from build123d import *

# Parameters (mm, degrees)
F1_DEPTH    = 15
F3_DEPTH    = 65
F4_T1_DEPTH = 15
F4_T3_DEPTH = 80
F4_T8_DEPTH = 80


# Not quite as in the source:
# - a fillet or chamfer that OpenCascade refuses, or shapes differently, is made with other operations: its cross-section is extruded or revolved along the edge and cut away or added
# - a feature names something its author has since deleted; it is built from what else it names


with BuildPart() as f1:
    # F0 (on Top) → F1 (new body)
    with BuildSketch(Plane.XY):
        Polygon((0, 88), (0, 0), (18, 0), (18, 5), (14, 5), (14, 4), (4, 4), (4, 84), (14, 84), (17, 81), (27, 81), (27, 85), (18.6568542495, 85), (15.6568542495, 88), align=None)
    extrude(amount=F1_DEPTH)

    # F2 (on face) → F3 (join)
    with BuildSketch(Plane.XY.offset(15)):
        Polygon((4, 10), (0, 10), (0, 0), (18, 0), (18, 5), (14, 5), (14, 4), (4, 4), align=None)
    extrude(amount=F3_DEPTH)

    # F4: chamfer of 2.5 on 3 edges, made by hand

    # F4_s2 → F4_t1 (join)
    with BuildSketch(Plane.XY):
        Polygon((6.5, 84), (4, 81.5), (4, 84), align=None)
    extrude(amount=F4_T1_DEPTH)

    # F4_s4 → F4_t3 (join)
    with BuildSketch(Plane.XY):
        Polygon((4, 6.5), (6.5, 4), (4, 4), align=None)
    extrude(amount=F4_T3_DEPTH)


with BuildPart() as f4_tool6:
    # F4_s7 → F4_t8 (new body)
    with BuildSketch(Plane.XY):
        Polygon((11.5, 4), (14, 6.5), (14, 4), align=None)
    extrude(amount=F4_T8_DEPTH)

    split(bisect_by=Plane.XZ.offset(-5), keep=Keep.TOP)


with BuildPart() as f1_1:
    add(f1.part)

    # F4_t5: union F4_tool6
    add(f4_tool6.part)


solid = f1_1.part
Geometry: final body of the model. Coordinates: model frame, mm. A direction names the side the tool comes from. Give positions to 0.01 mm unless a question says otherwise; leave off trailing zeros. Loops run counter-clockwise (first coordinate to the right, second up) from the corner with the lowest first, then second, coordinate; pieces in that order, holes last. Notation, with made-up numbers: M 44,-30.75 L 75,-30.75 A15 ccw 75,-13.75 Z; hole C -14,-8 d4. An arc over 180 degrees is marked long. Put each result on its own line as item: value.
1) Reachability of faces 1 (the flat face through (15, 5, 41)), 2 (the flat face through (23, 85, 7)), 3 (the flat face through (2, 10, 47)) from +Z, -Z, +X, -X, +Y, -Y: full face, straight path, thin tool, end or side. Return the list, or none.
Computed values:
face 1: +Z, -Z, +X
face 2: +Z, -Z, +X, +Y
face 3: +Z, +X, -X, +Y
2) Cut plane B-B, the plane x = 7.5. Return the cut outline in (y, z).
Computed values:
outline: M 0,0 L 4,0 L 4,80 L 0,80 Z; M 84,0 L 88,0 L 88,15 L 84,15 Z
3) Cut plane D-D, the plane z = 16.5. Return the cut outline in (x, y).
Computed values:
outline: M 0,0 L 18,0 L 18,5 L 12.5,5 L 11.5,4 L 6.5,4 L 4,6.5 L 4,10 L 0,10 Z
4) Mould query, pull axis Y, two halves, no side actions, for faces 4 (the flat face through (10, 84, 7)), 5 (the flat face through (7, 3, 80)), 6 (the flat face through (8, 88, 7)). Classes: released by +Y, released by -Y, zero draft, split by the parting line, or undercut.
Computed values:
face 4: undercut
face 5: zero draft
face 6: released by +Y
5) Cut plane C-C, the plane y = 66. Return the cut outline in (x, z).
Computed values:
outline: M 0,0 L 4,0 L 4,15 L 0,15 Z
6) Material intervals for L1, parallel to Y at x = 10.5, z = 7; L2, parallel to Y at x = 12.75, z = 49; L3, parallel to Z at x = 1.75, y = 78.5, sorted ascending. Write a range as from..to.
Computed values:
L1: y = 0..4, 84..88
L2: y = 0..5
L3: z = 0..15
7) First-contact query: P1, Ø3, axis at x = 3, z = 51, coming from the +Y side; P2, Ø1.5, axis at y = 2, z = 22, coming from the +X side; P3, Ø6.5, axis at x = 23, z = 8.5, coming from the +Y side. Flat tips, straight axial feed; report the tip coordinate or a pass-through.
Computed values:
P1: stops at y = 10
P2: stops at x = 18
P3: stops at y = 85
8) Cut plane A-A, the plane z = 6. Return the cut outline in (x, y).
Computed values:
outline: M 0,0 L 18,0 L 18,5 L 12.5,5 L 11.5,4 L 6.5,4 L 4,6.5 L 4,81.5 L 6.5,84 L 14,84 L 17,81 L 27,81 L 27,85 L 18.66,85 L 15.66,88 L 0,88 Z
